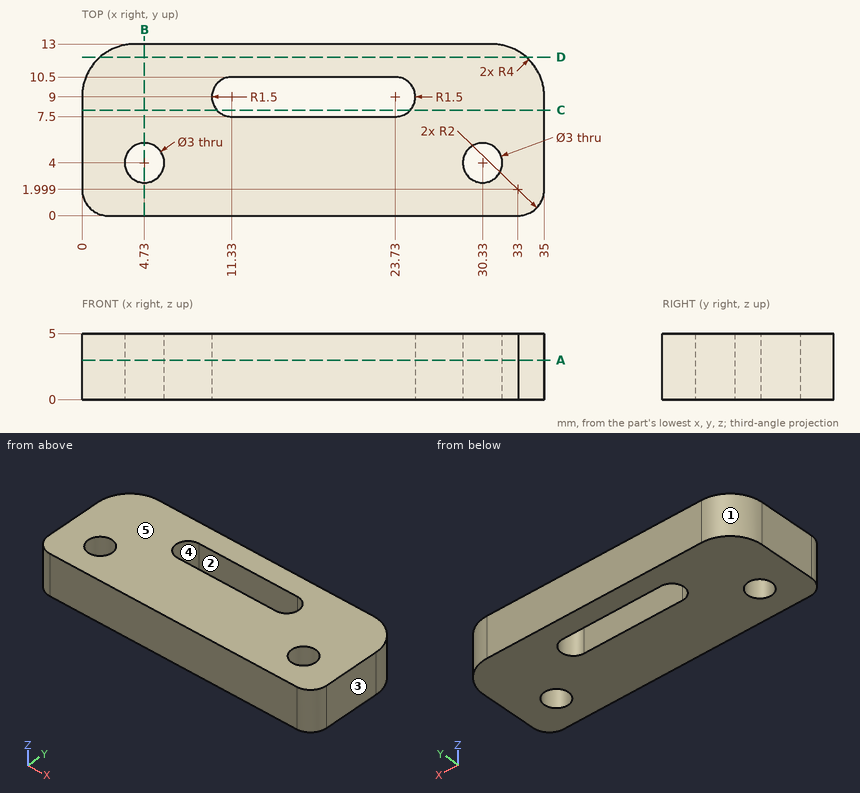
Design review of the part shown in the three views and the two pictorial views. Dimensions are in mm from the part's minimum x, y and z. A direction names the side the tool comes from. Round coordinates to 2 decimals unless told otherwise and drop trailing zeros. Write each loop counter-clockwise with the first axis right and the second up, starting at its lowest first coordinate (ties: lowest second). Pieces come first, ordered by that corner, then holes. Notation, with made-up numbers: M 52.25,-14 L 104.25,-14 A21 cw 104.25,6 Z; hole C 7.5,-2 d6. An arc over 180 degrees is marked long. One line per item, written item: value. Start each with the question number.
1. For the marked faces 4 and 5, list the 3-axis set-ups (+Z, -Z, +X, -X, +Y, -Y) from which the entire face can be reached by the end or side of a thin tool; tool diameter is ignored.
2. Take a section at B-B on x = 4.73. State the section outline as (y, z) points.
3. Clearance check with flat-ended pins moving along their axes: P1, Ø2.5, axis at x = 4.73, y = 4, coming from the -Z side; P2, Ø1.5, axis at y = 4, z = 3.5, coming from the -X side. State where each tip first meets the part, or that it passes through.
4. Take a section at D-D on y = 12. State the section outline as (x, z) points, then the cut area to 3 significant figures.
5. Take a section at A-A on z = 3. State the section outline as (x, y) points.
6. To check wall thickness, follow probe 1 along Y at (x, z) = (18.5, 1.5); probe 2 along Y at (x, z) = (30.33, 3.1); probe 3 along X at (y, z) = (9.25, 1.8). State the ranges of each line that lie inside material, in increasing order. Write a range as from..to.
7. Take a section at C-C on y = 8. State the section outline as (x, z) points.
8. Draft analysis for pull direction X (two halves, no side actions). For the marked faces 1, 2 and 3, state which applies: pulls with the +X half, pulls with the -X half, needs draft (parallel to the pull), parting line crosses it, or undercut.
Computed:
1. face 4: +Z, -Z
1. face 5: +Z, +X, -X, +Y, -Y
2. outline: M 0,0 L 2.5,0 L 2.5,5 L 0,5 Z; M 5.5,0 L 13,0 L 13,5 L 5.5,5 Z
3. P1: passes through
3. P2: stops at x = 0
4. outline: M 1.35,0 L 33.65,0 L 33.65,5 L 1.35,5 Z
4. area: 161 mm²
5. outline: M 0,2 A2 ccw 2,0 L 33.06,0 A2 ccw 35,2 L 35,9 A4 ccw 31,13 L 4,13 A4 ccw 0,9 Z; hole C 4.73,4 d3; hole M 11.33,7.5 L 23.73,7.5 A1.5 ccw 23.73,10.5 L 11.33,10.5 A1.5 ccw Z; hole C 30.33,4 d3
6. probe 1: y = 0..7.5, 10.5..13
6. probe 2: y = 0..2.5, 5.5..13
6. probe 3: x = 0.01..9.85, 25.21..34.99
7. outline: M 0,0 L 10.21,0 L 10.21,5 L 0,5 Z; M 24.85,0 L 35,0 L 35,5 L 24.85,5 Z
8. face 1: pulls with the -X half
8. face 2: undercut
8. face 3: pulls with the +X half
